Build history of the part. All positions in model axes, mm. A direction names the side the tool comes from. Round coordinates to 2 decimals unless told otherwise and drop trailing zeros. Order: outer loops, then holes, each group sorted by start corner. A loop starts at its lowest first (then second) coordinate and runs counter-clockwise, first axis right, second up. Notation, with made-up numbers: (-24, 47.5) - (-20, 47.5) arc R26 ccw to (-20, 74.5) - close; hole circle Ø10 at (-8, 73.5). An arc over 180 degrees is marked (long way). Write each question's results on one line, items separated by ' | '. Start each with the question number.
```python
from build123d import *

# Parameters (mm, degrees)
SKETCH1_R           = 6.35
BOSS_EXTRUDE1_DEPTH = 12.7
SKETCH2_R           = 1.7
CUT_EXTRUDE1_DEPTH  = 6.35
CUT_EXTRUDE2_DEPTH  = 6.35
SKETCH4_W           = 3.114007597
SKETCH4_H           = 7.898709862
CUT_EXTRUDE3_DEPTH  = 14.224
SKETCH5_R           = 1.27
CUT_EXTRUDE4_DEPTH  = 3.81


with BuildPart() as part:
    # Sketch1 → Boss-Extrude1 (new body)
    with BuildSketch(Plane.XY):
        Circle(SKETCH1_R)
    extrude(amount=BOSS_EXTRUDE1_DEPTH)

    # Sketch2 → Cut-Extrude1 (cut)
    with BuildSketch(Plane.XY.offset(12.7)):
        Circle(SKETCH2_R)
    extrude(amount=-CUT_EXTRUDE1_DEPTH, mode=Mode.SUBTRACT)

    # Sketch3 → Cut-Extrude2 (cut)
    with BuildSketch(Plane(origin=(0, 0, 0), x_dir=(-1, 0, 0), z_dir=(0, 0, -1))):
        Polygon((-2.646216495, -1.536512804), (0.007550874, -3.05994711), (2.653767369, -1.523434307), (2.646216495, 1.536512804), (-0.007550874, 3.05994711), (-2.653767369, 1.523434307), align=None)
    extrude(amount=-CUT_EXTRUDE2_DEPTH, mode=Mode.SUBTRACT)

    # Sketch4 → Cut-Extrude3 (cut)
    with BuildSketch(Plane(origin=(0, 0, 0), x_dir=(-1, 0, 0), z_dir=(0, 0, -1))):
        with Locations((-6.6621984, 0.173181196)):
            Rectangle(SKETCH4_W, SKETCH4_H)
    extrude(amount=-CUT_EXTRUDE3_DEPTH, mode=Mode.SUBTRACT)

    # Sketch5 → Cut-Extrude4 (cut)
    with BuildSketch(Plane(origin=(5.105194602, 0, 0), x_dir=(0, 0, -1), z_dir=(1, 0, 0))):
        with Locations((-10.668, 0)):
            Circle(SKETCH5_R)
        with Locations((-2.032, 0)):
            Circle(SKETCH5_R)
    extrude(amount=-CUT_EXTRUDE4_DEPTH, mode=Mode.SUBTRACT)


solid = part.part
```
1. Cut at D-D (z = 2). List the corners of the cut face in (x, y).
2. Flat gauge pins, fed straight in: pin 1 Ø3 at (x, z) = (-5, 7.5) entering from -Y; pin 2 Ø1 at (x, z) = (1, 4) entering from -Y. Where does each tip first touch, or does it go through?
3. Cut at B-B (y = 0). List the corners of the cut face in (x, z).
4. 3-axis set-ups, long thin cutter, end or side, ignore diameter. For faces 4 (the face through (3.227, 0.056, 11.937)), 5 (the face through (-2, 0, 12.7)), 6 (the face through (1.312, 2.302, 3.131)): which of +Z, -Z, +X, -X, +Y, -Y reach the whole face in a straight line?
5. Cut at C-C (y = -2.25). List the corners of the cut face in (x, z), plus the area to 3 significant figures.
6. Cut at A-A (z = 6). List the corners of the cut face in (x, y).
7. Wall check: line 1 (Z direction, x = 4.3, y = 0); line 2 (Y direction, x = 0, z = 8.25); line 3 (Y direction, x = 2.5, z = 0.75). Give the ranges that are in metal, low to high. Write a range as from..to.
8. Mould opens along X. For faces 1 (the face through (5.105, 0, 6)), 2 (the face through (3.89, -0.77, 3.04)), 3 (the face through (2, 0, 6.35)) say: pulls with the +X half, pulls with the -X half, needs draft (parallel to the pull), parting line crosses it, or undercut.
A:
1) outline: (-2.65, -1.52) - (-2.65, 1.54) - (0.01, 3.06) - (2.65, 1.52) - (2.65, 1.27) - (5.11, 1.27) - (5.11, 3.78) arc R6.35 ccw (long way) to (5.11, -3.78) - (5.11, -1.27) - (2.65, -1.27) - (2.65, -1.54) - (-0.01, -3.06) - close
2) pin 1: stops at y = -5.3 | pin 2: stops at y = -6.33
3) outline: (-6.35, 0) - (-2.65, 0) - (-2.65, 6.35) - (-1.7, 6.35) - (-1.7, 12.7) - (-6.35, 12.7) - close; (1.7, 6.35) - (2.65, 6.35) - (2.65, 3.3) - (5.11, 3.3) - (5.11, 9.4) - (1.7, 9.4) - close; (1.7, 11.94) - (5.11, 11.94) - (5.11, 12.7) - (1.7, 12.7) - close; (2.65, 0) - (5.11, 0) - (5.11, 0.76) - (2.65, 0.76) - close
4) face 4: +X | face 5: +Z, +X, -X, +Y, -Y | face 6: -Z
5) outline: (-5.94, 0) - (-1.4, 0) - (-1.4, 6.35) - (1.4, 6.35) - (1.4, 0) - (5.11, 0) - (5.11, 12.7) - (-5.94, 12.7) - close | area: 122 mm^2
6) outline: (5.11, -3.78) - (5.11, 3.78) arc R6.35 ccw (long way) to start; hole (-2.65, -1.52) - (-0.01, -3.06) - (2.65, -1.54) - (2.65, 1.52) - (0.01, 3.06) - (-2.65, 1.54) - close
7) line 1: z = 0..0.76, 3.3..9.4, 11.94..12.7 | line 2: y = -6.35..-1.7, 1.7..6.35 | line 3: y = -5.84..-1.62, 1.61..5.84
8) face 1: pulls with the +X half | face 2: needs draft | face 3: undercut
